For this review, take the finished solid that the model builds, in its own axes (mm). Round coordinates to 2 decimals unless told otherwise and drop trailing zeros. Order: outer loops, then holes, each group sorted by start corner. A loop starts at its lowest first (then second) coordinate and runs counter-clockwise, first axis right, second up. Notation, with made-up numbers: (10.5, 55) - (61.5, 55) arc R16 ccw to (61.5, 78) - close; hole circle Ø6 at (-3, 23.5). An arc over 180 degrees is marked (long way). One line per item, written item: value.
```python
from build123d import *

# Parameters (mm, degrees)
F0_R         = 7.7216
F1_DEPTH     = 6.35
F2_T1_DEPTH  = 46.447303982
F2_T3_DEPTH  = 46.447303982
F2_T5_DEPTH  = 46.447303982
F2_T7_DEPTH  = 46.447303982
F2_T9_DEPTH  = 46.447303982
F2_T11_DEPTH = 46.447303982
F2_T14_ANGLE = 299.426156199
F2_T16_ANGLE = 299.426156199
F2_T18_ANGLE = 299.426156199
F2_T20_ANGLE = 299.426156199
F2_T22_ANGLE = 299.426156199
F2_T24_ANGLE = 299.426156199


# Not quite as in the source:
# - a fillet or chamfer that OpenCascade refuses, or shapes differently, is made with other operations: its cross-section is extruded or revolved along the edge and cut away or added


with BuildPart() as f1:
    # F0 (on Front) → F1 (new body)
    with BuildSketch(Plane.XZ):
        with BuildLine():
            Line((-22.9108, 2.227330358), (-38.1, -24.0811357684))
            Line((-38.1, -24.0811357684), (-7.7216, -24.0811357684))
            ThreePointArc((-7.7216, -24.0811357684), (0, -16.3595357684), (7.7216, -24.0811357684))
            Line((7.7216, -24.0811357684), (38.1, -24.0811357684))
            Line((38.1, -24.0811357684), (22.9108, 2.227330358))
            ThreePointArc((22.9108, 2.227330358), (12.3628982421, 5.0536321158), (15.1892, 15.6015338737))
            Line((15.1892, 15.6015338737), (0, 41.91))
            Line((0, 41.91), (-15.1892, 15.6015338737))
            ThreePointArc((-15.1892, 15.6015338737), (-12.3628982421, 12.7752321158), (-11.3284, 8.9144321158))
            ThreePointArc((-11.3284, 8.9144321158), (-15.1892, 2.227330358), (-22.9108, 2.227330358))
        make_face()
        with Locations((-21.6022160579, -14.5561357684)):
            Circle(F0_R, mode=Mode.SUBTRACT)
        with Locations((21.6022160579, -14.5561357684)):
            Circle(F0_R, mode=Mode.SUBTRACT)
        Circle(F0_R, mode=Mode.SUBTRACT)
        with Locations((0, 22.86)):
            Circle(F0_R, mode=Mode.SUBTRACT)
    extrude(amount=F1_DEPTH)

    # F2: chamfer of 3.1242 on 18 edges, made by hand

    # F2_s2 → F2_t1 (cut)
    with BuildSketch(Plane(origin=(-0.7460116682, 0, -1.2921301124), x_dir=(0, 1, 0), z_dir=(-0.5, 0, -0.8660254038))):
        Polygon((-6.35, -17.8308), (-3.2258, -20.955), (-6.35, -20.955), align=None)
        Polygon((-3.1242, -20.955), (0, -17.8308), (0, -20.955), align=None)
    extrude(amount=F2_T1_DEPTH, mode=Mode.SUBTRACT)

    # F2_s4 → F2_t3 (cut)
    with BuildSketch(Plane(origin=(22.1647883318, 0, 38.3905395297), x_dir=(0, 1, 0), z_dir=(-0.5, 0, -0.8660254038))):
        Polygon((-6.35, -17.8308), (-3.2258, -20.955), (-6.35, -20.955), align=None)
        Polygon((-3.1242, -20.955), (0, -17.8308), (0, -20.955), align=None)
    extrude(amount=F2_T3_DEPTH, mode=Mode.SUBTRACT)

    # F2_s6 → F2_t5 (cut)
    with BuildSketch(Plane(origin=(1.0588636592, 0, -1.834005656), x_dir=(0, 1, 0), z_dir=(-0.5, 0, 0.8660254038))):
        Polygon((-6.35, -17.8308), (-3.2258, -20.955), (-6.35, -20.955), align=None)
        Polygon((0, -17.8308), (-3.1242, -20.955), (0, -20.955), align=None)
    extrude(amount=F2_T5_DEPTH, mode=Mode.SUBTRACT)

    # F2_s8 → F2_t7 (cut)
    with BuildSketch(Plane(origin=(23.9696636592, 0, -41.5166752981), x_dir=(0, 1, 0), z_dir=(-0.5, 0, 0.8660254038))):
        Polygon((-6.35, -17.8308), (-3.2258, -20.955), (-6.35, -20.955), align=None)
        Polygon((0, -17.8308), (-3.1242, -20.955), (0, -20.955), align=None)
    extrude(amount=F2_T7_DEPTH, mode=Mode.SUBTRACT)

    # F2_s10 → F2_t9 (cut)
    with BuildSketch(Plane.YZ.offset(-0.312851991)):
        Polygon((-6.35, -20.9569357684), (-3.2258, -24.0811357684), (-6.35, -24.0811357684), align=None)
        Polygon((-3.1242, -24.0811357684), (0, -20.9569357684), (0, -24.0811357684), align=None)
    extrude(amount=F2_T9_DEPTH, mode=Mode.SUBTRACT)

    # F2_s12 → F2_t11 (cut)
    with BuildSketch(Plane.YZ.offset(-46.134451991)):
        Polygon((-6.35, -20.9569357684), (-3.2258, -24.0811357684), (-6.35, -24.0811357684), align=None)
        Polygon((-3.1242, -24.0811357684), (0, -20.9569357684), (0, -24.0811357684), align=None)
    extrude(amount=F2_T11_DEPTH, mode=Mode.SUBTRACT)

    # F2_s13 → F2_t14 (revolve, cut)
    with BuildSketch(Plane(origin=(-0.0451180595, 0, 9.0096042642), x_dir=(0, 1, 0), z_dir=(-0.0050077109, 0, 0.9999874613))):
        Polygon((-6.35, 29.8509202393), (-3.2258, 26.7267202393), (-6.35, 26.7267202393), align=None)
    revolve(axis=Axis((-19.05, -6.35, 8.9144321158), (0, -1, 0)), revolution_arc=F2_T14_ANGLE, mode=Mode.SUBTRACT)

    # F2_s15 → F2_t16 (revolve, cut)
    with BuildSketch(Plane(origin=(0.0451180595, 0, 9.0096042642), x_dir=(0, 1, 0), z_dir=(0.0050077109, 0, 0.9999874613))):
        Polygon((-3.2258, -26.7267202393), (-6.35, -29.8509202393), (-6.35, -26.7267202393), align=None)
    revolve(axis=Axis((19.05, -6.35, 8.9144321158), (0, 1, 0)), revolution_arc=F2_T16_ANGLE, mode=Mode.SUBTRACT)

    # F2_s17 → F2_t18 (revolve, cut)
    with BuildSketch(Plane(origin=(10.4872096098, 0, -6.1250197631), x_dir=(0, 1, 0), z_dir=(0.8635106895, 0, -0.5043305355))):
        Polygon((-6.35, -31.6401181517), (-3.2258, -28.5159181517), (-6.35, -28.5159181517), align=None)
    revolve(axis=Axis((0, -6.35, -24.0811357684), (0, 1, 0)), revolution_arc=F2_T18_ANGLE, mode=Mode.SUBTRACT)

    # F2_s19 → F2_t20 (revolve, cut)
    with BuildSketch(Plane(origin=(10.4872096098, 0, -6.1250197631), x_dir=(0, 1, 0), z_dir=(0.8635106895, 0, -0.5043305355))):
        Polygon((-3.1242, -28.5159181517), (0, -31.6401181517), (0, -28.5159181517), align=None)
    revolve(axis=Axis((0, 0, -24.0811357684), (0, 1, 0)), revolution_arc=F2_T20_ANGLE, mode=Mode.SUBTRACT)

    # F2_s21 → F2_t22 (revolve, cut)
    with BuildSketch(Plane(origin=(0.0451180595, 0, 9.0096042642), x_dir=(0, 1, 0), z_dir=(0.0050077109, 0, 0.9999874613))):
        Polygon((-3.1242, -26.7267202393), (0, -29.8509202393), (0, -26.7267202393), align=None)
    revolve(axis=Axis((19.05, 0, 8.9144321158), (0, 1, 0)), revolution_arc=F2_T22_ANGLE, mode=Mode.SUBTRACT)

    # F2_s23 → F2_t24 (revolve, cut)
    with BuildSketch(Plane(origin=(-10.5323276693, 0, -6.0107202694), x_dir=(0, 1, 0), z_dir=(-0.8685184004, 0, -0.4956569258))):
        Polygon((-3.1242, -24.9062127584), (0, -28.0304127584), (0, -24.9062127584), align=None)
    revolve(axis=Axis((-19.05, 0, 8.9144321158), (0, 1, 0)), revolution_arc=F2_T24_ANGLE, mode=Mode.SUBTRACT)


solid = f1.part
```
Item 1: Take a section at C-C (x = 5). Count the separate pieces of the cut face and the enclosed holes in it, plus the area to 3 significant figures.
Returned:
separate pieces: 3
enclosed holes: 0
area: 147 mm^2
Item 2: The part is to be moulded in two halves that separate along X. For faces 1 (the flat face through (22.698, -4.463, -22.844)), 2 (the flat face through (-29.33, -4.46, -11.36)), 3 (the cylindrical face through (-1.67, -3.13, 15.32)), say which applies: +X half, -X half, draft (parallel to the pull), parting line (faces both ways), or undercut.
Returned:
face 1: draft
face 2: -X half
face 3: undercut
Item 3: For P1, Ø1, axis at y = -1, z = 22.5, coming from the +X side; P2, Ø3, axis at x = -3, z = 5.5, coming from the +Y side; P3, Ø14, axis at x = -21.6, z = -14.56, coming from the -Y side; P4, Ø2, axis at x = 0.5, y = -5.5, coming from the +Z side, all flat-tipped, find the tip position at first contact; note any pin that passes through.
Returned:
P1: x = 9.4
P2: y = 0
P3: through
P4: z = 39.09
Item 4: Take a section at B-B (y = -1.5). Write out the cut boundary in (x, z).
Returned:
outline: (-35.29, -22.46) - (-9.2, -22.46) arc R9.35 cw to (9.2, -22.46) - (35.29, -22.46) - (22.25, 0.13) arc R9.35 cw to (13.04, 16.07) - (0, 38.66) - (-13.04, 16.07) arc R9.35 cw to (-22.25, 0.13) - close; hole circle Ø15.44 at (-21.6, -14.56); hole circle Ø15.44 at (0, 0); hole circle Ø15.44 at (0, 22.86); hole circle Ø15.44 at (21.6, -14.56)
Item 5: Wall thickness on line 1 (X direction, y = -2.75, z = -12); line 2 (Z direction, x = 7, y = -4.75); line 3 (X direction, y = -3.5, z = -12.5): over which ranges is each line inside the solid? List them lowest first.
Returned:
line 1: -30.69 to -28.89, -14.32 to 14.32, 28.89 to 30.69
line 2: -18.04 to -3.26, 3.26 to 19.6, 26.12 to 26.74
line 3: -31.1 to -29.05, -14.16 to 14.16, 29.05 to 31.1
Item 6: Take a section at A-A (x = -19.05). Write out the cut boundary in (y, z).
Returned:
outline: (-6.35, -7.27) - (0, -7.27) - (0, -1.93) - (-3.12, 1.19) - (-3.23, 1.19) - (-6.35, -1.93) - close; (-5.46, -21.84) - (-3.23, -24.08) - (-3.12, -24.08) - (-0.89, -21.84) - close
